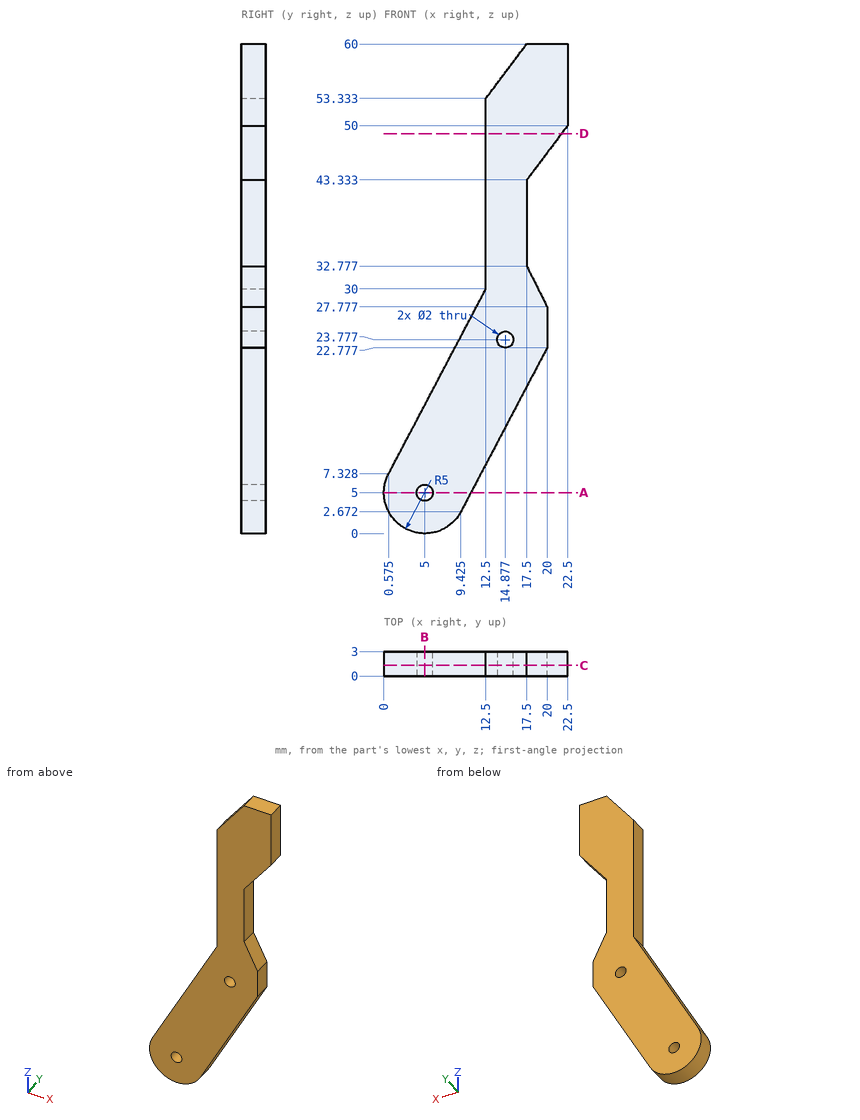
Can you work these out from the drawing? Everything is in mm from the part's minimum corner. Coordinates: 2 decimals unless noted, no trailing zeros. Write each loop counter-clockwise with the first axis right and the second up, starting at its lowest first coordinate (ties: lowest second). Pieces come first, ordered by that corner, then holes. Notation, with made-up numbers: (0.25, 68) -> (43.25, 68) arc R21 cw to (43.25, 74) -> close; hole circle Ø6 at (62, -25.75). An arc over 180 degrees is marked (long way). Write each question's results on one line, items separated by ' | '. Start each with the question number.
Q1. Imagine slicing it at C-C (y = 1.3). Write out the boundary of the cut face in (x, z) (1 decimal).
Q2. Imagine slicing it at D-D (z = 49). Write out the boundary of the cut face in (x, y).
Q3. I'm going to push a flat-ended pin straight in: pin 1 (1.2 mm diameter, centred on x = 5, z = 5, fed in from -Y). Where does the tip first touch, or does it pass through?
Q4. Imagine slicing it at B-B (x = 5). Write out the boundary of the cut face in (y, z).
Q5. If I drill on probe 1 along X at (y, z) = (2.75, 52.5); probe 2 along Z at (x, y) = (4.25, 0.6) (1 decimal); probe 3 along Z at (x, y) = (15, 1.9) (1 decimal), over which ranges is the centre line in solid material (lowest first)?
Q6. Imagine slicing it at A-A (z = 5). Write out the boundary of the cut face in (x, y).
Taken from the geometry:
1) outline: (0.6, 7.3) arc R5 ccw to (9.4, 2.7) -> (20, 22.8) -> (20, 27.8) -> (17.5, 32.8) -> (17.5, 43.3) -> (22.5, 50) -> (22.5, 60) -> (17.5, 60) -> (12.5, 53.3) -> (12.5, 30) -> close; hole circle Ø2 at (5, 5); hole circle Ø2 at (14.9, 23.8)
2) outline: (12.5, 0) -> (21.75, 0) -> (21.75, 3) -> (12.5, 3) -> close
3) pin 1: passes through
4) outline: (0, 0) -> (3, 0) -> (3, 4) -> (0, 4) -> close; (0, 6) -> (3, 6) -> (3, 15.74) -> (0, 15.74) -> close
5) probe 1: x = 12.5 to 22.5 | probe 2: z = 0.1 to 4.3, 5.7 to 14.3 | probe 3: z = 13.3 to 22.8, 24.8 to 56.7
6) outline: (0, 0) -> (4, 0) -> (4, 3) -> (0, 3) -> close; (6, 0) -> (10.65, 0) -> (10.65, 3) -> (6, 3) -> close
